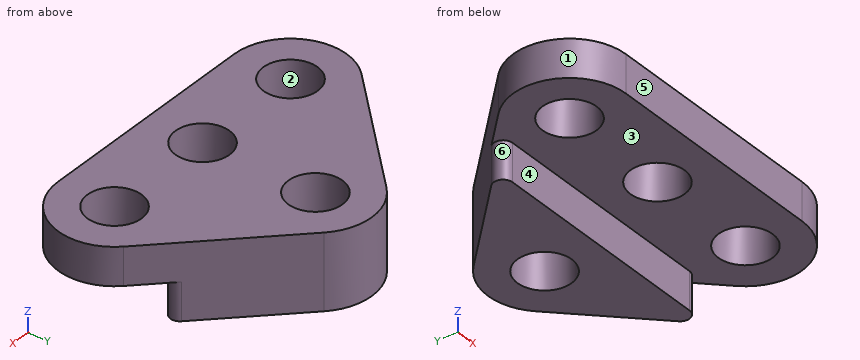
from build123d import *

# Parameters (mm, degrees)
SKETCH1_R           = 2.286
SKETCH1_R_2         = 2.2859999999999996
BOSS_EXTRUDE1_DEPTH = 3.175
BOSS_EXTRUDE2_START = -3.175
SKETCH1_4_R         = 2.2859999999999996
BOSS_EXTRUDE2_DEPTH = 3.175
FILLET1_R           = 0.79375


with BuildPart() as part:
    # Sketch1 → Boss-Extrude1 (new body)
    with BuildSketch(Plane.XY):
        with BuildLine():
            Line((-12.89259604540093, 3.3675960454009313), (-3.367596045400929, 12.892596045400932))
            ThreePointArc((-3.367596045400929, 12.892596045400932), (2.89e-15, 14.287499999999998), (3.3675960454009344, 12.892596045400932))
            Line((3.3675960454009344, 12.892596045400932), (12.892596045400932, 3.3675960454009357))
            ThreePointArc((12.892596045400932, 3.3675960454009357), (13.924976273585006, -1.8225298466387372), (9.525, -4.762499999999998))
            Line((9.525, -4.762499999999998), (-9.525, -4.7625))
            ThreePointArc((-9.525, -4.7625), (-13.924976273585003, -1.8225298466387385), (-12.89259604540093, 3.3675960454009313))
        make_face()
        Circle(SKETCH1_R, mode=Mode.SUBTRACT)
        with Locations((-9.525, 0)):
            Circle(SKETCH1_R, mode=Mode.SUBTRACT)
        with Locations((9.525, 3.5e-15)):
            Circle(SKETCH1_R, mode=Mode.SUBTRACT)
        with Locations((2.6e-15, 9.525)):
            Circle(SKETCH1_R_2, mode=Mode.SUBTRACT)
    extrude(amount=BOSS_EXTRUDE1_DEPTH)

    # Sketch1_4 → Boss-Extrude2 (add)
    with BuildSketch(Plane.XY.offset(BOSS_EXTRUDE2_START)):
        with BuildLine():
            Line((-3.367596045400928, 12.892596045400932), (-11.49769209080186, 4.762500000000003))
            Line((-11.49769209080186, 4.762500000000004), (11.497692090801866, 4.762500000000003))
            Line((11.497692090801866, 4.762500000000002), (3.3675960454009335, 12.892596045400932))
            ThreePointArc((3.3675960454009344, 12.892596045400932), (2.66e-15, 14.287499999999998), (-3.367596045400929, 12.892596045400932))
        make_face()
        with Locations((2.6e-15, 9.525)):
            Circle(SKETCH1_4_R, mode=Mode.SUBTRACT)
    extrude(amount=BOSS_EXTRUDE2_DEPTH)

    # Fillet1
    fillet1_edges = [part.edges().sort_by_distance(p)[0] for p in [
        (11.497692090801866, 4.762500000000003, -1.5875),
        (-11.49769209080186, 4.762500000000003, -1.5875),
    ]]
    fillet(fillet1_edges, radius=FILLET1_R)


solid = part.part
The model under review builds one solid part; all positions refer to its coordinate system, in mm. Face numbers are marked on the shaded views. A direction names the side the tool comes from. Give positions to 0.01 mm unless a question says otherwise; leave off trailing zeros. Order: outer loops, then holes, each group sorted by start corner. A loop starts at its lowest first (then second) coordinate and runs counter-clockwise, first axis right, second up. Notation, with made-up numbers: M -3,35 L 30,35 A13 ccw 30,45 Z; hole C 29,60.5 d3. An arc over 180 degrees is marked long. One line per question, with ' | ' between items. Start each with the question number.
1) Consider section D-D, the plane z = -2.5. Give the boundary of the cut face in (x, y) (1 decimal).
2) For the marked faces 4, 5 and 6, list the 3-axis set-ups (+Z, -Z, +X, -X, +Y, -Y) from which the entire face can be reached by the end or side of a thin tool; tool diameter is ignored.
3) Clearance check with flat-ended pins moving along their axes: P1, Ø1, axis at x = 8, y = 9.5, coming from the -Z side; P2, Ø1, axis at x = 2.5, z = -2.5, coming from the -Y side; P3, Ø5.5, axis at x = 0, y = 9.525, coming from the -Z side (3 decimals); P4, Ø1.5, axis at y = 12.5, z = 2, coming from the +X side. State where each tip first meets the part, or that it passes through.
4) Consider section C-C, the plane x = 8.5. Give the boundary of the cut face in (y, z) (1 decimal), then the cut area to 3 significant figures.
5) Mouldability with a two-part tool opening along Y and no side actions: class the marked faces 1, 2 and 3 as pulls with the +Y half, pulls with the -Y half, needs draft (parallel to the pull), parting line crosses it, or undercut.
6) Wall thickness on L1, parallel to Y at x = 0, z = 1.7; L2, parallel to Y at x = -1, z = 1; L3, parallel to X at y = 1.25, z = 1: over which ranges is each line inside the solid? List them lowest first. Write a range as from..to.
7) Consider section A-A, the plane x = 0. Give the boundary of the cut face in (y, z) (1 decimal).
8) Consider section B-B, the plane y = 0. Give the boundary of the cut face in (x, z) (1 decimal), then the cut area to 3 significant figures.
Found:
1) outline: M -10.1,6.1 A0.8 ccw -9.6,4.8 L 9.6,4.8 A0.8 ccw 10.1,6.1 L 3.4,12.9 A4.8 ccw -3.4,12.9 Z; hole C 0,9.5 d4.6
2) face 4: -Z, +X, -X, -Y | face 5: +Z, -Z, +X, -X, -Y | face 6: -Z, -X
3) P1: passes through | P2: stops at y = 4.76 | P3: stops at z = -3.175 | P4: stops at x = 4.51
4) outline: M -4.8,0 L -2,0 L -2,3.2 L -4.8,3.2 Z; M 2,0 L 4.8,0 L 4.8,-3.2 L 7.8,-3.2 L 7.8,3.2 L 2,3.2 Z | area: 36.3 mm²
5) face 1: parting line crosses it | face 2: undercut | face 3: needs draft
6) L1: y = -4.76..-2.29, 2.29..7.24, 11.81..14.29 | L2: y = -4.76..-2.06, 2.06..7.47, 11.58..14.18 | L3: x = -14.12..-11.44, -7.61..-1.91, 1.91..7.61, 11.44..14.12
7) outline: M -4.8,0 L -2.3,0 L -2.3,3.2 L -4.8,3.2 Z; M 2.3,0 L 4.8,0 L 4.8,-3.2 L 7.2,-3.2 L 7.2,3.2 L 2.3,3.2 Z; M 11.8,-3.2 L 14.3,-3.2 L 14.3,3.2 L 11.8,3.2 Z
8) outline: M -14.3,0 L -11.8,0 L -11.8,3.2 L -14.3,3.2 Z; M -7.2,0 L -2.3,0 L -2.3,3.2 L -7.2,3.2 Z; M 2.3,0 L 7.2,0 L 7.2,3.2 L 2.3,3.2 Z; M 11.8,0 L 14.3,0 L 14.3,3.2 L 11.8,3.2 Z | area: 47.2 mm²
